```python
from build123d import *

# Parameters (mm, degrees)
BOSS_EXTRUDE1_DEPTH = 38.1
SKETCH2_R           = 11.049
CUT_EXTRUDE1_DEPTH  = 6.35
SKETCH2_4_R         = 3.556
CUT_EXTRUDE2_DEPTH  = 6.35
SKETCH4_W           = 94.447991824
SKETCH4_H           = 31.75
CUT_EXTRUDE5_DEPTH  = 76.2


with BuildPart() as part:
    # Sketch1 → Boss-Extrude1 (new body)
    with BuildSketch(Plane.XY):
        Polygon((0, 76.2), (0, 0), (6.35, 0), (6.35, 69.85), (6.35, 76.2), align=None)
        Polygon((88.097991824, 76.2), (6.35, 76.2), (6.35, 69.85), (94.447991824, 69.85), (94.447991824, 101.6), (88.097991824, 101.6), align=None)
    extrude(amount=BOSS_EXTRUDE1_DEPTH)

    # Sketch2 → Cut-Extrude1 (cut)
    with BuildSketch(Plane.ZY):
        with Locations((19.05, 20.32)):
            Circle(SKETCH2_R)
    extrude(amount=-CUT_EXTRUDE1_DEPTH, mode=Mode.SUBTRACT)

    # Sketch2_4 → Cut-Extrude2 (cut)
    with BuildSketch(Plane.ZY):
        with Locations((19.05, 42.672)):
            Circle(SKETCH2_4_R)
    extrude(amount=-CUT_EXTRUDE2_DEPTH, mode=Mode.SUBTRACT)

    # Sketch4 → Cut-Extrude5 (cut)
    with BuildSketch(Plane.XY.offset(38.1)):
        with Locations((47.223995912, 85.725)):
            Rectangle(SKETCH4_W, SKETCH4_H)
    extrude(amount=-CUT_EXTRUDE5_DEPTH, mode=Mode.SUBTRACT)


solid = part.part
```
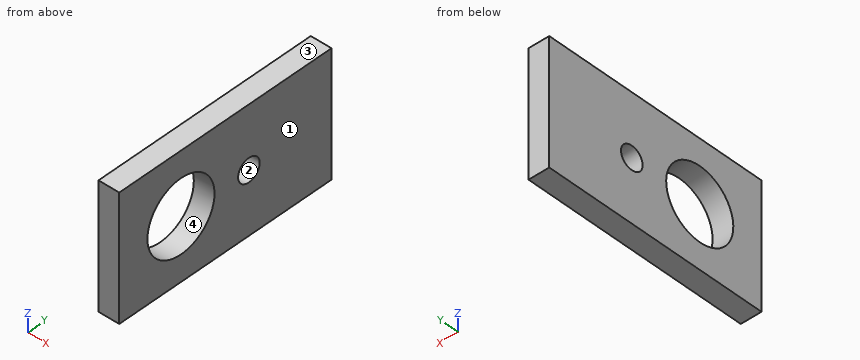
Geometry: final body of the model. Coordinates: model frame, mm. Face numbers are marked on the shaded views. Coordinates: 2 decimals unless noted, no trailing zeros. Order: outer loops, then holes, each group sorted by start corner. A loop starts at its lowest first (then second) coordinate and runs counter-clockwise, first axis right, second up. Notation, with made-up numbers: (-10, 8) - (31, 8) arc R21 cw to (31, 28) - close; hole circle Ø6 at (20, -7). An arc over 180 degrees is marked (long way). Return JSON: item names as keys, results as strings. Group by question number.
1. Cut plane B-B (y = 20.32). Output: boundary loops of the cut face in (x, z).
2. Material intervals for line 1 along Y through (x, z) = (1.75, 19.05); line 2 along Y through (x, z) = (1.5, 22); line 3 along Y through (x, z) = (2.75, 25), sorted ascending. Write a range as [from, to].
3. Pull-direction query (Z, two-part tool) for the marked faces 1, 2, 3 and 4; classes: pulls with the +Z half, pulls with the -Z half, needs draft (parallel to the pull), parting line crosses it, or undercut.
4. Pin query (flat end, axial travel): pin 1 (2 mm diameter, centred on y = 29, z = 15.5, fed in from -X). Return the tip coordinate at first contact, or that it passes through.
5. Cut plane C-C (x = 3.5). Output: boundary loops of the cut face in (y, z).
6. Cut plane A-A (z = 19.05). Output: boundary loops of the cut face in (x, y).
Resolved:
{
 "1": {"outline": "(0, 0) - (6.35, 0) - (6.35, 8) - (0, 8) - close; (0, 30.1) - (6.35, 30.1) - (6.35, 38.1) - (0, 38.1) - close"},
 "2": {"line 1": "y = [0, 9.27], [31.37, 39.12], [46.23, 69.85]", "line 2": "y = [0, 9.67], [30.97, 40.69], [44.66, 69.85]", "line 3": "y = [0, 11.01], [29.63, 69.85]"},
 "3": {"face 1": "needs draft", "face 2": "undercut", "face 3": "pulls with the +Z half", "face 4": "undercut"},
 "4": {"pin 1": "passes through"},
 "5": {"outline": "(0, 0) - (69.85, 0) - (69.85, 38.1) - (0, 38.1) - close; hole circle Ø22.1 at (20.32, 19.05); hole circle Ø7.11 at (42.67, 19.05)"},
 "6": {"outline": "(0, 0) - (6.35, 0) - (6.35, 9.27) - (0, 9.27) - close; (0, 31.37) - (6.35, 31.37) - (6.35, 39.12) - (0, 39.12) - close; (0, 46.23) - (6.35, 46.23) - (6.35, 69.85) - (0, 69.85) - close"}
}
